Source: CAD feature listing. Evaluate the final solid. Frame: model axes, mm. A direction names the side the tool comes from. Round coordinates to 2 decimals unless told otherwise and drop trailing zeros. Order: outer loops, then holes, each group sorted by start corner. A loop starts at its lowest first (then second) coordinate and runs counter-clockwise, first axis right, second up. Notation, with made-up numbers: M 61.5,-2.5 L 96.5,-2.5 A18 ccw 96.5,22.5 Z; hole C -21.75,33.25 d5. An arc over 180 degrees is marked long. Answer in a Markdown table with one row per item. Add a question column.
Solid Edge part; units mm, degrees
sketch "Sketch1" plane through (0, 0, 0) normal (0, 0, 1) x (1, 0, 0)
  line L0 (0, 0) -> (42.5, 0)
  line L1 (42.5, 0) -> (42.5, 80)
  line L2 (42.5, 80) -> (0, 80)
  line L3 (0, 80) -> (0, 0)
extrude "Protrusion1" add sketch "Sketch1" along normal blind 1
sketch "Sketch2" plane through (21.25, 40, 1) normal (0, 0, 1) x (1, 0, 0)
  line L0 (-20, 40) -> (-20, -40)
  line L1 (-20, -40) -> (20, -40)
  line L2 (20, -40) -> (20, 40)
  line L3 (20, 40) -> (-20, 40)
extrude "Vysunutí_2" add sketch "Sketch2" along normal blind 1
sketch "Sketch3" plane through (21.25, 40, 2) normal (0, 0, 1) x (1, 0, 0)
  line L0 (-22.5, -40) -> (22.5, -40)
  line L1 (22.5, -40) -> (22.5, 40)
  line L2 (22.5, 40) -> (-22.5, 40)
  line L3 (-22.5, 40) -> (-22.5, -40)
extrude "Vysunutí_3" add sketch "Sketch3" along normal blind 1
sketch "Sketch4" plane through (21.25, 40, 3) normal (0, 0, 1) x (1, 0, 0)
  line L0 (-22.5, 75) -> (-22.5, 40)
  line L1 (-22.5, 40) -> (22.5, 40)
  line L2 (22.5, 40) -> (-12.5, 75)
  line L3 (-22.5, 75) -> (-12.5, 75)
extrude "Protrusion2" add sketch "Sketch4" against normal blind 16
sketch "Sketch5" plane through (21.25, 57.5, 3) normal (0, 0, 1) x (0, -1, 0)
  line L0 (-23.75, 21.25) -> (-23.75, -22.5)
  line L1 (-23.75, -22.5) -> (-57.5, -22.5)
  line L2 (-57.5, -22.5) -> (-57.5, -12.5)
  line L3 (-57.5, -12.5) -> (-23.75, 21.25)
extrude "Cutout1" cut sketch "Sketch5" against normal blind 15
sketch "Sketch6" plane through (21.25, 97.5, -13) normal (0, 0, -1) x (0, -1, 0)
  line L0 (-15, 12.5) -> (-7.6278, 5.1278)
  line L1 (-7.6278, 5.1278) -> (16.25, -18.75)
  line L2 (17.5, -20) -> (16.25, -18.75)
  line L3 (17.5, 22.5) -> (17.5, -20)
  line L4 (16.25, 22.5) -> (17.5, 22.5)
  line L5 (16.25, 22.5) -> (-15, 22.5)
  line L6 (-17.5, 22.5) -> (-15, 22.5)
  line L7 (-17.5, 15) -> (-17.5, 22.5)
  line L8 (-15, 12.5) -> (-17.5, 15)
extrude "Vysunutí_6" add sketch "Sketch6" along normal blind 1
sketch "Sketch7" plane through (20, 96.25, -14) normal (0, 0, -1) x (-1, 0, 0)
  line L0 (21.25, 16.25) -> (21.25, 17.5)
  line L1 (21.25, 18.75) -> (21.25, 17.5)
  line L2 (12.25, 18.75) -> (21.25, 18.75)
  line L3 (11, 17.5) -> (12.25, 18.75)
  line L4 (9.75, 16.25) -> (11, 17.5)
  line L5 (9.75, 16.25) -> (-22.75, -16.25)
  line L6 (-22.75, -16.25) -> (-21.25, -16.25)
  line L7 (21.25, -16.25) -> (-21.25, -16.25)
  line L8 (21.25, 16.25) -> (21.25, -16.25)
extrude "Vysunutí_7" add sketch "Sketch7" along normal blind 1
(1) Cut plane C-C (z = -4.25). Return loops of the section in (x, y), and give its area (3 significant figures).
(2) Access query for faces 1 (the face through (21, 41, 0)), 2 (the face through (25.495, 97.255, -14.493)), 3 (the face through (23.99, 97.26, -13.49)). Directions: +Z, -Z, +X, -X, +Y, -Y. A direction counts if a zero-diameter tool reaches every point of the face in a straight line with its end or side. Return the directions, or none.
(3) Pin query (flat end, axial travel): pin 1 (0.8 mm diameter, centred on x = 42.5, y = 57.5, fed in from -Z); pin 2 (5 mm diameter, centred on x = 20, z = -3.5, fed in from -Y); pin 3 (4.5 mm diameter, centred on x = 13.5, z = -7.5, fed in from +Y); pin 4 (3 mm diameter, centred on y = 77.5, z = -6, fed in from -X). Return the tip coordinate at first contact, or that it passes through.
(4) Draft query along Z for faces 4 (the face through (21, 0, 1)), 5 (the face through (21, 41, 3)), 6 (the face through (26, 96, -14)), 7 (the face through (0, 41, 2)). Return one class per face: +Z half, -Z half, draft (parallel to the pull), parting line (faces both ways), or undercut.
(5) Line query: line 1 (Z direction, x = 20, y = 41.5); line 2 (X direction, y = 52, z = 0.5); line 3 (Y direction, x = 39, z = -4.25). Output: solid intervals per line, ascending. Write a range as from..to.
(6) Cut plane A-A (x = 26.5). Return loops of the section in (y, z).
(7) Cut plane B-B (y = 26). Return loops of the section in (x, z), and give its area (4 significant figures).
(8) Cut plane D-D (x = 5). Return loops of the section in (y, z), and give its area (3 significant figures).
Answer list:
| question | item | result |
|---|---|---|
| 1 | outline | M -1.25,80 L 43.75,80 L 42.5,81.25 L -1.25,81.25 Z |
| 1 | area | 55.5 mm² |
| 2 | face 1 | -Z, +X, -X, -Y |
| 2 | face 2 | -Z, +X, +Y |
| 2 | face 3 | +X, +Y |
| 3 | pin 1 | z = 0 |
| 3 | pin 2 | y = 80 |
| 3 | pin 3 | y = 81.25 |
| 3 | pin 4 | through |
| 4 | face 4 | draft |
| 4 | face 5 | +Z half |
| 4 | face 6 | undercut |
| 4 | face 7 | undercut |
| 5 | line 1 | 0..3 |
| 5 | line 2 | 0..42.5 |
| 5 | line 3 | 80..81.25 |
| 6 | outline | M 0,0 L 80,0 L 80,-15 L 96.25,-15 L 96.25,-14 L 94.75,-14 L 94.75,-13 L 97.25,-13 L 97.25,-12 L 81.25,-12 L 81.25,3 L 0,3 Z |
| 7 | outline | M -1.25,2 L 1.25,2 L 1.25,1 L 0,1 L 0,0 L 42.5,0 L 42.5,1 L 41.25,1 L 41.25,2 L 43.75,2 L 43.75,3 L -1.25,3 Z |
| 7 | area | 127.5 mm² |
| 8 | outline | M 0,0 L 80,0 L 80,-15 L 115,-15 L 115,-12 L 81.25,-12 L 81.25,3 L 0,3 Z |
| 8 | area | 364 mm² |
